```python
from build123d import *

# Parameters (mm, degrees)
SKETCH1_W           = 26
SKETCH1_H           = 26
SKETCH1_W_2         = 5
SKETCH1_H_2         = 43
SKETCH1_R           = 2.5
BOSS_EXTRUDE1_DEPTH = 17
CHAMFER1_SIZE       = 2.5


with BuildPart() as part:
    # Sketch1 → Boss-Extrude1 (new body)
    # profile 1 of 4: a face of its own
    with BuildSketch(Plane.XY):
        Rectangle(SKETCH1_W, SKETCH1_H)
    # profile 2 of 4: a face of its own
    with BuildSketch(Plane.XY):
        Polygon((-2.5, -23), (2.5, -23), (13, -23), (13, -13), (-13, -13), (-13, -23), align=None)
    # profile 3 of 4: a face of its own
    with BuildSketch(Plane.XY):
        with Locations((0, -44.5)):
            Rectangle(SKETCH1_W_2, SKETCH1_H_2)
    # profile 4 of 4: a face of its own
    with BuildSketch(Plane.XY):
        Polygon((6.5, -70), (6.5, -75), (2.5, -79), (-2.5, -79), (-6.5, -75), (-6.5, -70), (-2.5, -66), (2.5, -66), align=None)
        with Locations((0, -72.5)):
            Circle(SKETCH1_R, mode=Mode.SUBTRACT)
    extrude(amount=BOSS_EXTRUDE1_DEPTH)

    # Chamfer1
    chamfer1_edges = [part.edges().sort_by_distance(p)[0] for p in [
        (-13, 13, 8.5),
        (13, 13, 8.5),
        (13, -23, 8.5),
        (2.5, -23, 8.5),
        (-2.5, -23, 8.5),
        (-13, -23, 8.5),
    ]]
    chamfer(chamfer1_edges, length=CHAMFER1_SIZE)


solid = part.part
```
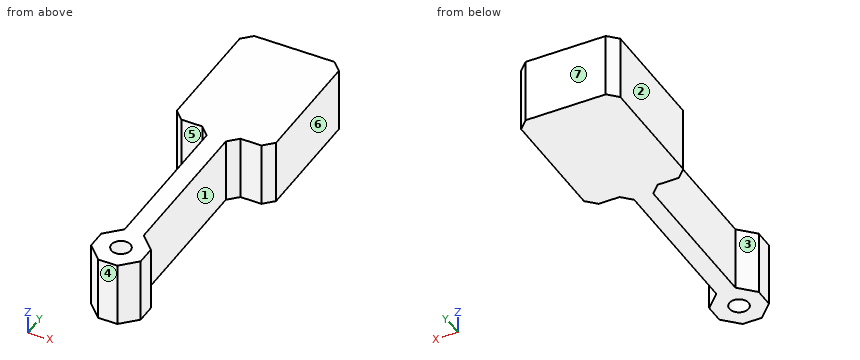
The model under review builds one solid part; all positions refer to its coordinate system, in mm. Face numbers are marked on the shaded views. A direction names the side the tool comes from. Coordinates: 2 decimals unless noted, no trailing zeros. Order: outer loops, then holes, each group sorted by start corner. A loop starts at its lowest first (then second) coordinate and runs counter-clockwise, first axis right, second up. Notation, with made-up numbers: (-38, -9.75) -> (-19, -9.75) arc R9 cw to (-19, -4.75) -> close; hole circle Ø3 at (68.5, 30.25). An arc over 180 degrees is marked (long way). Answer in a Markdown table with one row per item. Add a question column.
Item 1: We need section D-D on x = 11.75. Write out the cut boundary in (y, z).
Item 2: Mouldability with a two-part tool opening along Y and no side actions: class the marked faces 4, 5, 6 and 7 as +Y half, -Y half, draft (parallel to the pull), parting line (faces both ways), or undercut.
Item 3: We need section A-A on y = -72.5. Write out the cut boundary in (x, z), plus the area to 3 significant figures.
Item 4: Clearance check with flat-ended pins moving along their axes: pin 1 (4 mm diameter, centred on y = -73.5, z = 9.5, fed in from +X); pin 2 (8 mm diameter, centred on y = -31, z = 3, fed in from -X); pin 3 (1.6 mm diameter, centred on x = -7.5, z = 9.5, fed in from -Y); pin 4 (1.5 mm diameter, centred on x = -8.5, y = -0.5, fed in from -Z). State where each tip first meets the part, or that it passes through.
Item 5: We need section C-C on z = 2.5. Write out the cut boundary in (x, y), plus the area to 3 significant figures.
Item 6: We need section B-B on x = 0. Write out the cut boundary in (y, z), plus the area to 3 significant figures.
Item 7: To check wall thickness, follow probe 1 along Y at (x, z) = (0, 11.25); probe 2 along Y at (x, z) = (0.5, 12.25); probe 3 along Y at (x, z) = (-10, 3). State the ranges of each line that lie inside material, in increasing order.
Item 8: Machinability: for the marked faces 1, 2 and 3, which of the approach directions +Z, -Z, +X, -X, +Y, -Y give a long, thin tool a straight path to every point of the face, cutting with its end or side? Answer none if there is none.
Final values:
| question | item | result |
|---|---|---|
| 1 | outline | (-21.75, 0) -> (11.75, 0) -> (11.75, 17) -> (-21.75, 17) -> close |
| 2 | face 4 | -Y half |
| 2 | face 5 | undercut |
| 2 | face 6 | draft |
| 2 | face 7 | +Y half |
| 3 | outline | (-6.5, 0) -> (-2.5, 0) -> (-2.5, 17) -> (-6.5, 17) -> close; (2.5, 0) -> (6.5, 0) -> (6.5, 17) -> (2.5, 17) -> close |
| 3 | area | 136 mm2 |
| 4 | pin 1 | stops at x = 6.5 |
| 4 | pin 2 | stops at x = -2.5 |
| 4 | pin 3 | stops at y = -23 |
| 4 | pin 4 | stops at z = 0 |
| 5 | outline | (-13, -20.5) -> (-10.5, -23) -> (-5, -23) -> (-2.5, -25.5) -> (-2.5, -66) -> (-6.5, -70) -> (-6.5, -75) -> (-2.5, -79) -> (2.5, -79) -> (6.5, -75) -> (6.5, -70) -> (2.5, -66) -> (2.5, -25.5) -> (5, -23) -> (10.5, -23) -> (13, -20.5) -> (13, 10.5) -> (10.5, 13) -> (-10.5, 13) -> (-13, 10.5) -> close; hole circle Ø5 at (0, -72.5) |
| 5 | area | 1,260 mm2 |
| 6 | outline | (-79, 0) -> (-75, 0) -> (-75, 17) -> (-79, 17) -> close; (-70, 0) -> (13, 0) -> (13, 17) -> (-70, 17) -> close |
| 6 | area | 1,480 mm2 |
| 7 | probe 1 | y = -79 to -75, -70 to 13 |
| 7 | probe 2 | y = -79 to -74.95, -70.05 to 13 |
| 7 | probe 3 | y = -23 to 13 |
| 8 | face 1 | +Z, -Z, +X |
| 8 | face 2 | +Z, -Z, -X, +Y, -Y |
| 8 | face 3 | +Z, -Z, -X |
